```python
from build123d import *

# Parameters (mm, degrees)
BOSS_EXTRUDE1_DEPTH = 12.7
CUT_EXTRUDE2_DEPTH  = 6.35
CUT_EXTRUDE3_DEPTH  = 571.619829491
FILLET1_R           = 3.175
SKETCH7_W           = 110.518116872
SKETCH7_H           = 6.5
CUT_EXTRUDE4_DEPTH  = 6.35


with BuildPart() as part:
    # Sketch1 → Boss-Extrude1 (new body)
    with BuildSketch(Plane.XY):
        Polygon((-524.529885057, -25.691954023), (75.470114943, -25.691954023), (75.470114943, 224.308045977), (-391.864893443, 224.308045977), (-524.529885057, 24.308045977), align=None)
    extrude(amount=BOSS_EXTRUDE1_DEPTH)

    # Sketch4 → Cut-Extrude2 (cut)
    with BuildSketch(Plane.XY):
        Polygon((-519.529885057, 22.800489254), (-519.529885057, -20.691954023), (70.470114943, -20.691954023), (70.470114943, 219.308045977), (-389.181518234, 219.308045977), align=None)
        Polygon((-513.029885057, 20.840665514), (-513.029885057, -14.191954023), (63.970114943, -14.191954023), (63.970114943, 212.808045977), (-385.693130461, 212.808045977), align=None, mode=Mode.SUBTRACT)
    extrude(amount=CUT_EXTRUDE2_DEPTH, mode=Mode.SUBTRACT)

    # Sketch6 → Cut-Extrude3 (cut, through all)
    with BuildSketch(Plane(origin=(0, 0, 0), x_dir=(-1, 0, 0), z_dir=(0, 0, -1))):
        Polygon((443.734064292, 125.308045977), (435.400730959, 119.780337993), (448.114459322, 100.613671326), (456.447792655, 106.14137931), (460.614459322, 108.905233302), (447.900730959, 128.071899969), align=None)
    extrude(amount=-CUT_EXTRUDE3_DEPTH, mode=Mode.SUBTRACT)

    # Fillet1
    fillet1_edges = [part.edges().sort_by_distance(p)[0] for p in [
        (-447.900730959, 128.071899969, 9.525),
        (-460.614459322, 108.905233302, 9.525),
        (-435.400730959, 119.780337993, 6.35),
        (-448.114459322, 100.613671326, 6.35),
    ]]
    fillet(fillet1_edges, radius=FILLET1_R)

    # Sketch7 → Cut-Extrude4 (cut)
    with BuildSketch(Plane(origin=(0, 0, 0), x_dir=(-1, 0, 0), z_dir=(0, 0, -1))):
        with Locations((-36.124416508, 216.058045977)):
            Rectangle(SKETCH7_W, SKETCH7_H)
    extrude(amount=-CUT_EXTRUDE4_DEPTH, mode=Mode.SUBTRACT)


solid = part.part
```
Design review of the part built by this model. Coordinates are the model's own, in mm. A direction names the side the tool comes from. Give positions to 0.01 mm unless a question says otherwise; leave off trailing zeros. Write each loop counter-clockwise with the first axis right and the second up, starting at its lowest first coordinate (ties: lowest second). Pieces come first, ordered by that corner, then holes. Notation, with made-up numbers: (44, -18.5) -> (97, -18.5) arc R17 cw to (97, -3.5) -> close; hole circle Ø7 at (19, -22.75). An arc over 180 degrees is marked (long way). Answer in a Markdown table with one row per item.
(1) Mouldability with a two-part tool opening along X and no side actions: class faces 4 (the flat face through (-524.53, 0, 6)), 5 (the flat face through (-229, 101, 0)), 6 (the flat face through (-484.34, 64.09, 3.13)) as +X half, -X half, draft (parallel to the pull), parting line (faces both ways), or undercut.
Results:
| item | result |
|---|---|
| face 4 | -X half |
| face 5 | draft |
| face 6 | undercut |
(2) Consider section B-B (x = 23.5). State the section outline as (y, z) points, then the cut area to 3 significant figures.
Results:
| item | result |
|---|---|
| outline | (-25.69, 0) -> (-20.69, 0) -> (-20.69, 6.35) -> (-14.19, 6.35) -> (-14.19, 0) -> (212.81, 0) -> (212.81, 6.35) -> (219.31, 6.35) -> (219.31, 0) -> (224.31, 0) -> (224.31, 12.7) -> (-25.69, 12.7) -> close |
| area | 3,090 mm2 |
(3) To check wall thickness, follow probe 1 along Y at (x, z) = (-134, 1); probe 2 along X at (y, z) = (18, 2.5); probe 3 along X at (y, z) = (21, 3.5). State the ranges of each line that lie inside material, in increasing order.
Results:
| item | result |
|---|---|
| probe 1 | -25.69 to -20.69, -14.19 to 212.81, 219.31 to 224.31 |
| probe 2 | -524.53 to -519.53, -513.03 to 63.97, 70.47 to 75.47 |
| probe 3 | -524.53 to -519.53, -512.92 to 63.97, 70.47 to 75.47 |
(4) For faces 1 (the flat face through (-226, 220, 0)), 2 (the flat face through (-441.693, 110.294, 6.261)), 3 (the flat face through (-453.443, 122.43, 3.131)), list the 3-axis set-ups (+Z, -Z, +X, -X, +Y, -Y) from which the entire face can be reached by the end or side of a thin tool; tool diameter is ignored.
Results:
| item | result |
|---|---|
| face 1 | -Z, +X, -X, +Y, -Y |
| face 2 | +Z, -Z |
| face 3 | -Z |
(5) Consider section C-C (y = 181). State the section outline as (x, z) points, then the cut area to 3 significant figures.
Results:
| item | result |
|---|---|
| outline | (-420.59, 0) -> (-414.59, 0) -> (-414.59, 6.35) -> (-406.79, 6.35) -> (-406.79, 0) -> (63.97, 0) -> (63.97, 6.35) -> (70.47, 6.35) -> (70.47, 0) -> (75.47, 0) -> (75.47, 12.7) -> (-420.59, 12.7) -> close |
| area | 6,210 mm2 |
(6) Clearance check with flat-ended pins moving along their axes: pin 1 (5 mm diameter, centred on y = 153.5, z = 2.5, fed in from -X); pin 2 (1.5 mm diameter, centred on y = 91, z = 9, fed in from -X). State where each tip first meets the part, or that it passes through.
Results:
| item | result |
|---|---|
| pin 1 | x = -440.49 |
| pin 2 | x = -480.79 |
